The listing builds one solid part. Answer for the finished solid, in the listing's coordinates (mm). Face numbers are marked on the shaded views. A direction names the side the tool comes from. Coordinates: 2 decimals unless noted, no trailing zeros. Order: outer loops, then holes, each group sorted by start corner. A loop starts at its lowest first (then second) coordinate and runs counter-clockwise, first axis right, second up. Notation, with made-up numbers: (65.25, -5.5) - (119.25, -5.5) arc R13 cw to (119.25, -0.5) - close; hole circle Ø2 at (22, 58). An arc over 180 degrees is marked (long way). One line per item, written item: value. Start each with the question number.
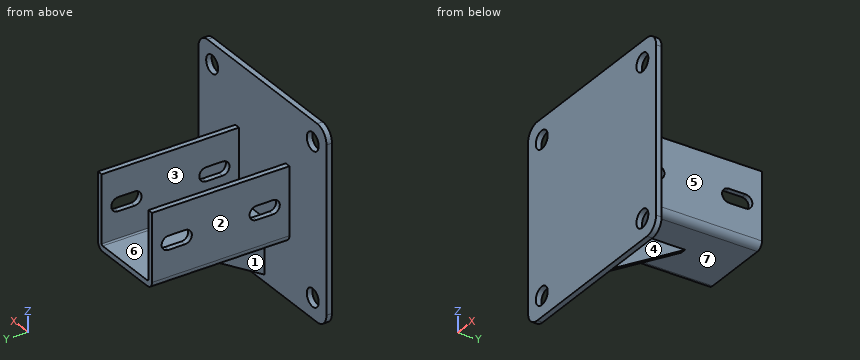
```python
from build123d import *

# Parameters (mm, degrees)
SKETCH_2_W          = 140
SKETCH_2_H          = 140
EXTRUDE_1_DEPTH     = 4
EXTRUDE_1_2_DEPTH   = 100
EXTRUDE_2_DEPTH     = 2
CUT_EXTRUDE_1_DEPTH = 100.5
SKETCH_6_R          = 6.5
CUT_EXTRUDE_2_DEPTH = 5
FILLET_1_R          = 10


with BuildPart() as part:
    # Эскиз2 → Extrude 1 (new body)
    with BuildSketch(Plane(origin=(0, 0, 0), x_dir=(1, 0, 0), z_dir=(0, 1, 0))):
        Rectangle(SKETCH_2_W, SKETCH_2_H)
    extrude(amount=EXTRUDE_1_DEPTH)

    # Эскиз3 → Extrude 1 2 (add)
    with BuildSketch(Plane(origin=(0, 4, 0), x_dir=(1, 0, 0), z_dir=(0, 1, 0))):
        with BuildLine():
            Line((-25.5, -25), (-25.5, 24))
            ThreePointArc((-25.5, 24), (-25.207106781, 24.707106781), (-24.5, 25))
            Line((-24.5, 25), (24.5, 25))
            ThreePointArc((24.5, 25), (25.207106781, 24.707106781), (25.5, 24))
            Line((25.5, 24), (25.5, -25))
            Line((25.5, -25), (29.5, -25))
            Line((29.5, -25), (29.5, 24))
            ThreePointArc((29.5, 24), (28.035533906, 27.535533906), (24.5, 29))
            Line((24.5, 29), (-24.5, 29))
            ThreePointArc((-24.5, 29), (-28.035533906, 27.535533906), (-29.5, 24))
            Line((-29.5, 24), (-29.5, -25))
            Line((-29.5, -25), (-25.5, -25))
        make_face()
    extrude(amount=EXTRUDE_1_2_DEPTH)

    # Эскиз4 → Бобышка-Вытянуть2 (add, symmetric)
    with BuildSketch(Plane(origin=(0, 0, 0), x_dir=(0, 0, -1), z_dir=(1, 0, 0))):
        Polygon((29, 66.353829072), (65, 4), (29, 4), align=None)
    extrude(amount=EXTRUDE_2_DEPTH, both=True)

    # Эскиз5 → Вырез-Вытянуть1 (cut, through all)
    with BuildSketch(Plane(origin=(29.5, 0, 0), x_dir=(0, 0, -1), z_dir=(1, 0, 0))):
        with BuildLine():
            Line((5, 92), (5, 80))
            ThreePointArc((5, 80), (0, 75), (-5, 80))
            Line((-5, 80), (-5, 92))
            ThreePointArc((-5, 92), (0, 97), (5, 92))
        make_face()
        with BuildLine():
            Line((5, 28), (5, 16))
            ThreePointArc((5, 16), (0, 11), (-5, 16))
            Line((-5, 16), (-5, 28))
            ThreePointArc((-5, 28), (0, 33), (5, 28))
        make_face()
    extrude(amount=-CUT_EXTRUDE_1_DEPTH, mode=Mode.SUBTRACT)

    # Эскиз6 → Вырез-Вытянуть2 (cut, through all)
    with BuildSketch(Plane(origin=(0, 4, 0), x_dir=(1, 0, 0), z_dir=(0, 1, 0))):
        with Locations(Location((-55, 55, 0), (0, 0, 270))):  # turned: the seam where the file's is
            Circle(SKETCH_6_R)
        with Locations(Location((-55, -55, 0), (0, 0, 270))):  # turned: the seam where the file's is
            Circle(SKETCH_6_R)
        with Locations(Location((55, 55, 0), (0, 0, 270))):  # turned: the seam where the file's is
            Circle(SKETCH_6_R)
        with Locations(Location((55, -55, 0), (0, 0, 270))):  # turned: the seam where the file's is
            Circle(SKETCH_6_R)
    extrude(amount=-CUT_EXTRUDE_2_DEPTH, mode=Mode.SUBTRACT)

    # Скругление1
    fillet_1_edges = [part.edges().sort_by_distance(p)[0] for p in [
        (70, 2, 70),
        (-70, 2, 70),
        (-70, 2, -70),
        (70, 2, -70),
    ]]
    fillet(fillet_1_edges, radius=FILLET_1_R)


solid = part.part
```
(1) The part is cut by section D-D on z = 19. Determine the outline of the cut face in (x, y).
(2) The part is cut by section B-B on x = 8. Determine the outline of the cut face in (y, z), plus the area to 3 significant figures.
(3) For a pull along X with two mould halves and no side action, classify the marked faces 5, 6 and 7 as pulls with the +X half, pulls with the -X half, needs draft (parallel to the pull), parting line crosses it, or undercut.
(4) The part is cut by section A-A on z = 53. Determine the outline of the cut face in (x, y), plus the area to 3 significant figures.
(5) Flat-ended cylindrical pins translate along their axes: pin 1 Ø1.5 at (x, z) = (44, 50.5) entering from -Y; pin 2 Ø8 at (x, y) = (6, 13) entering from +Z; pin 3 Ø1.2 at (x, y) = (28.5, 85.5) entering from +Z; pin 4 Ø6 at (y, z) = (53.5, 0) entering from -X. Find the tip coordinate at first contact, or state that the pin passes through.
(6) The part is cut by section C-C on y = 50. Determine the outline of the cut face in (x, z).
(7) Consider probe 1 along X at (y, z) = (2.2, -55); probe 2 along X at (y, z) = (45.5, 6); probe 3 along Y at (x, z) = (-32, -24.5). Determine where each line is inside the solid, lowest interval first.
(8) For the marked faces 1, 2, 3 and 4, determine the directions among +Z, -Z, +X, -X, +Y, -Y from which every point of the face is accessible in a straight line to the end or side of a thin tool.
Completed:
1. outline: (-70, 0) - (70, 0) - (70, 4) - (29.5, 4) - (29.5, 104) - (25.5, 104) - (25.5, 4) - (-25.5, 4) - (-25.5, 104) - (-29.5, 104) - (-29.5, 4) - (-70, 4) - close
2. outline: (0, -70) - (4, -70) - (4, -29) - (104, -29) - (104, -25) - (4, -25) - (4, 70) - (0, 70) - close
2. area: 960 mm2
3. face 5: pulls with the +X half
3. face 6: undercut
3. face 7: needs draft
4. outline: (-70, 0) - (-61.18, 0) - (-61.18, 4) - (-70, 4) - close; (-48.82, 0) - (48.82, 0) - (48.82, 4) - (-48.82, 4) - close; (61.18, 0) - (70, 0) - (70, 4) - (61.18, 4) - close
4. area: 461 mm2
5. pin 1: stops at y = 0
5. pin 2: stops at z = -25
5. pin 3: stops at z = 25
5. pin 4: stops at x = -29.5
6. outline: (-29.5, -24) arc R5 ccw to (-24.5, -29) - (-2, -29) - (-2, -38.44) - (2, -38.44) - (2, -29) - (24.5, -29) arc R5 ccw to (29.5, -24) - (29.5, 25) - (25.5, 25) - (25.5, -24) arc R1 cw to (24.5, -25) - (-24.5, -25) arc R1 cw to (-25.5, -24) - (-25.5, 25) - (-29.5, 25) - close
7. probe 1: x = -70 to -61.5, -48.5 to 48.5, 61.5 to 70
7. probe 2: x = -29.5 to -25.5, 25.5 to 29.5
7. probe 3: y = 0 to 4
8. face 1: -Z, -X, +Y
8. face 2: +Z, -Z, -X, +Y
8. face 3: +Z, +Y
8. face 4: -Z, +X, +Y
